For this review, take the finished solid that the model builds, in its own axes (mm). Face numbers are marked on the shaded views. Round coordinates to 2 decimals unless told otherwise and drop trailing zeros. Loops run counter-clockwise (first coordinate to the right, second up) from the corner with the lowest first, then second, coordinate; pieces in that order, holes last.
1) Mouldability with a two-part tool opening along X and no side actions: class the marked faces 1, 2 and 3 as pulls with the +X half, pulls with the -X half, needs draft (parallel to the pull), parting line crosses it, or undercut.
2) Wall thickness on L1, parallel to Y at x = 0, z = -9.1; L2, parallel to Y at x = 0, z = -3.5; L3, parallel to Z at x = -3.5, y = 0.25: over which ranges is each line inside the solid? List them lowest first.
3) Insertion check: pin 1 (5 mm diameter, centred on x = 0.5, y = -4.5, fed in from +Z); pin 2 (4 mm diameter, centred on x = 1, y = -2, fed in from +Z); pin 3 (1.5 mm diameter, centred on x = 3.5, z = 4, fed in from -Y); pin 4 (5 mm diameter, centred on y = 3.5, z = 2.5, fed in from -X). Each pin has a flat end and moves straight along its axis. Give the tip position at first contact, or say it passes through.
4) Take a section at A-A (z = 2.5). State the section outline as (x, y) points.
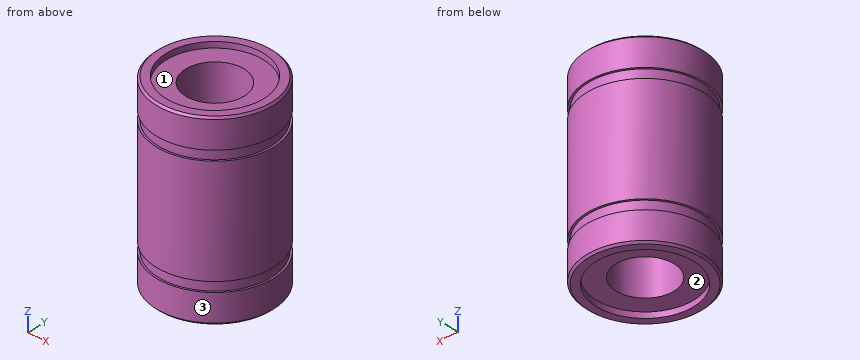
Autodesk Inventor part; units mm, degrees
ref_plane "YZ Plane" through (0, 0, 0) normal (1, 0, 0) x (0, 1, 0)
ref_plane "XZ Plane" through (0, 0, 0) normal (0, 1, 0) x (-1, 0, 0)
ref_plane "XY Plane" through (0, 0, 0) normal (0, 0, 1) x (1, 0, 0)
sketch "Эскиз1" plane through (0, 0, 0) normal (0, 0, 1) x (1, 0, 0)
  circle A0 centre (0, 0) radius 6
  dimension "d0" = 12
extrude "Выдавливание1" add sketch "Эскиз1" along normal mid plane 11
sketch "Эскиз2" plane through (0, 0, 5.5) normal (0, 0, 1) x (1, 0, 0)
  circle A0 centre (0, 0) radius 5.8
  dimension "d3" = 11.6
extrude "Выдавливание2" add sketch "Эскиз2" along normal blind 1
sketch "Эскиз3" plane through (0, 0, 6.5) normal (0, 0, 1) x (1, 0, 0)
  circle A0 centre (0, 0) radius 6
extrude "Выдавливание3" add sketch "Эскиз3" along normal blind 3
sketch "Эскиз4" plane through (0, 0, 9.5) normal (0, 0, 1) x (1, 0, 0)
  circle A0 centre (0, 0) radius 5
  dimension "d8" = 10
extrude "Выдавливание4" cut sketch "Эскиз4" against normal blind 0.6
sketch "Эскиз5" plane through (0, 0, 8.9) normal (0, 0, 1) x (1, 0, 0)
  circle A0 centre (0, 0) radius 3
  dimension "d11" = 6
extrude "Выдавливание5" cut sketch "Эскиз5" against normal through all
chamfer "Фаска1" distance 0.2 angle 45 1 edges at (-6, 0, 9.5)
mirror "Зеркальное отражение1" about plane through (0, 0, 0) normal (0, 0, 1) of "Выдавливание3", "Выдавливание4", "Выдавливание5", "Фаска1", "Выдавливание2"
properties part number "LM6UU" material "Сталь, нержавеющая, аустенитная"
Response:
1. face 1: undercut
1. face 2: undercut
1. face 3: parting line crosses it
2. L1: y = -6 to -5, 5 to 6
2. L2: y = -6 to -3, 3 to 6
2. L3: z = -8.9 to 8.9
3. pin 1: stops at z = 9.5
3. pin 2: stops at z = 8.9
3. pin 3: stops at y = -5.33
3. pin 4: stops at x = -5.92
4. outline: circle Ø12 at (0, 0); hole circle Ø6 at (0, 0)
